```python
from build123d import *

# Parameters (mm, degrees)
SKETCH1_W           = 12.7
SKETCH1_H           = 5.159375
BOSS_EXTRUDE1_DEPTH = 6.35
SKETCH2_R           = 0.5
BOSS_EXTRUDE2_DEPTH = 3.175
SKETCH3_R           = 0.9921875
CUT_EXTRUDE1_DEPTH  = 16.107337634


with BuildPart() as part:
    # Sketch1 → Boss-Extrude1 (new body)
    with BuildSketch(Plane(origin=(0, 0, 0), x_dir=(1, 0, 0), z_dir=(0, 1, 0))):
        with Locations((6.35, 2.5796875)):
            Rectangle(SKETCH1_W, SKETCH1_H)
    extrude(amount=BOSS_EXTRUDE1_DEPTH)

    # Sketch2 → Boss-Extrude2 (add)
    with BuildSketch(Plane.XZ):
        with Locations(Location((6.35, -2.5796875, 0), (0, 0, 270))):
            Circle(SKETCH2_R)
        with Locations(Location((1.5875, -2.5796875, 0), (0, 0, 270))):
            Circle(SKETCH2_R)
        with Locations(Location((11.1125, -2.5796875, 0), (0, 0, 270))):
            Circle(SKETCH2_R)
    extrude(amount=BOSS_EXTRUDE2_DEPTH)

    # Sketch3 → Cut-Extrude1 (cut, through all)
    with BuildSketch(Plane.XY):
        with Locations((9.525, 1)):
            Circle(SKETCH3_R)
        with Locations((3.175, 1)):
            Circle(SKETCH3_R)
    extrude(amount=-CUT_EXTRUDE1_DEPTH, mode=Mode.SUBTRACT)


solid = part.part
```
Can you work these out from the model? Positions are in its coordinate system, mm. A direction names the side the tool comes from. Give positions to 0.01 mm unless a question says otherwise; leave off trailing zeros. Loops run counter-clockwise (first coordinate to the right, second up) from the corner with the lowest first, then second, coordinate; pieces in that order, holes last. Notation, with made-up numbers: M 54.25,7.25 L 97.25,7.25 A8 cw 97.25,12.25 Z; hole C 86,-2 d2. An arc over 180 degrees is marked long. One line per item, written item: value.
(1) Suppose I cut it at D-D on x = 6.35. List the corners of the cut face in (y, z) for me (3 decimals).
Returned:
outline: M -3.175,-3.08 L 0,-3.08 L 0,-5.159 L 6.35,-5.159 L 6.35,0 L 0,0 L 0,-2.08 L -3.175,-2.08 Z
(2) Suppose I cut it at A-A on y = 1. List the corners of the cut face in (x, z) for me, plus the area to 3 significant figures.
Returned:
outline: M 0,-5.16 L 2.18,-5.16 L 2.18,0 L 0,0 Z; M 4.17,-5.16 L 8.53,-5.16 L 8.53,0 L 4.17,0 Z; M 10.52,-5.16 L 12.7,-5.16 L 12.7,0 L 10.52,0 Z
area: 45.0 mm^2
(3) I need wall thicknesses on line 1 (Y direction, x = 11.5, z = -4.6); line 2 (Y direction, x = 2.5, z = -1.7); line 3 (Z direction, x = 1.75, y = -2.5). Which ranges of each line are inside material? Lowest first, please.
Returned:
line 1: 0 to 6.35
line 2: 0 to 0.27, 1.73 to 6.35
line 3: -3.05 to -2.11
(4) Will this pin go through, and if not, where does the flat tip stop? pin 1 (1.6 mm diameter, centred on x = 9.525, y = 1, fed in from +Z).
Returned:
pin 1: through
(5) We'd pull the mould along X, two halves only. Please class faces 3 (the face through (6, 3, -5.159)), 4 (the face through (8.738, 0.396, -2.544)), 5 (the face through (12.7, 3, -3)): released by +X, released by -X, zero draft, split by the parting line, or undercut.
Returned:
face 3: zero draft
face 4: undercut
face 5: released by +X
(6) Which directions (+Z, -Z, +X, -X, +Y, -Y) give clear straight access to the entire face, cutting with the end or side of a thin tool? Please do faces 1 (the face through (11.13, -1.57, -2.08)), 2 (the face through (6, 3, 0)).
Returned:
face 1: -Y
face 2: +Z, +X, -X, +Y, -Y
(7) Suppose I cut it at B-B on z = -3.35. List the corners of the cut face in (x, y) for me (3 decimals).
Returned:
outline: M 0,0 L 12.7,0 L 12.7,6.35 L 0,6.35 Z; hole C 3.175,1 d1.984; hole C 9.525,1 d1.984
(8) Suppose I cut it at C-C on x = 2.75. List the corners of the cut face in (y, z) for me, plus the area to 3 significant figures.
Returned:
outline: M 0,-5.16 L 0.1,-5.16 L 0.1,0 L 0,0 Z; M 1.9,-5.16 L 6.35,-5.16 L 6.35,0 L 1.9,0 Z
area: 23.5 mm^2
